Here's how the part is built. I have some questions about the finished solid (model axes, mm). Face numbers are marked on the shaded views. A direction names the side the tool comes from. Round coordinates to 2 decimals unless told otherwise and drop trailing zeros. Write each loop counter-clockwise with the first axis right and the second up, starting at its lowest first coordinate (ties: lowest second). Pieces come first, ordered by that corner, then holes. Notation, with made-up numbers: M 32,22 L 43,22 A26 ccw 43,46 Z; hole C 13,34 d10. An arc over 180 degrees is marked long. Write item = value, one per line. Start each with the question number.
(1) Will these pins go through, and if not, where does the flat tip stop? pin 1 Ø1 at (x, z) = (13.5, 1) entering from -Y; pin 2 Ø5 at (x, z) = (11, 3.5) entering from -Y; pin 3 Ø2 at (x, z) = (13, 0.5) entering from +Y.
(2) On a 3-axis mill with a long thin cutter (end or side, diameter ignored), from which of +Z, -Z, +X, -X, +Y, -Y can I reach the whole of each face in a straight line? I mean the marked faces 4 and 5. Say none if no direction works.
(3) I need wall thicknesses on line 1 along X through (y, z) = (-0.5, -4.25); line 2 along Z through (x, y) = (12.5, 0); line 3 along Z through (x, y) = (2.25, -1.5). Which ranges of each line are inside material? Lowest first, please.
(4) I want a section at B-B (x = 15). List the corners of the cut face in (y, z) for me, and give its area (3 significant figures).
(5) I want a section at A-A (z = 0). List the corners of the cut face in (x, y) for me.
(6) If we mould it in two halves opening along Z, with no side actions, what happens to the marked faces 1, 2 and 3? For each: released by +Z, released by -Z, zero draft, split by the parting line, or undercut.
```python
from build123d import *

# Parameters (mm, degrees)
CUT_EXTRUDE_1_DEPTH = 2.5
FILLET_1_R          = 0.3
CHAMFER_1_SIZE      = 1


with BuildPart() as part:
    # Эскиз1 → Повернуть1 (revolve)
    with BuildSketch(Plane.XY):
        Polygon((0, 0), (0, 5), (6, 5), (6, 3), (18, 3), (18, 0), align=None)
    revolve(axis=Axis((18, 0, 0), (-1, 0, 0)))

    # Эскиз2 → Вырез-Вытянуть1 (cut)
    with BuildSketch(Plane.ZY):
        Polygon((-1.443375673, 2.5), (-2.886751346, 0), (-1.443375673, -2.5), (1.443375673, -2.5), (2.886751346, 0), (1.443375673, 2.5), align=None)
    extrude(amount=-CUT_EXTRUDE_1_DEPTH, mode=Mode.SUBTRACT)

    # Скругление1
    fillet_1_edges = [part.edges().sort_by_distance(p)[0] for p in [
        (6, -3, 0),
        (0, -5, 0),
    ]]
    fillet(fillet_1_edges, radius=FILLET_1_R)

    # Фаска1
    chamfer_1_edges = [part.edges().sort_by_distance(p)[0] for p in [
        (18, -3, 0),
    ]]
    chamfer(chamfer_1_edges, length=CHAMFER_1_SIZE)


solid = part.part
```
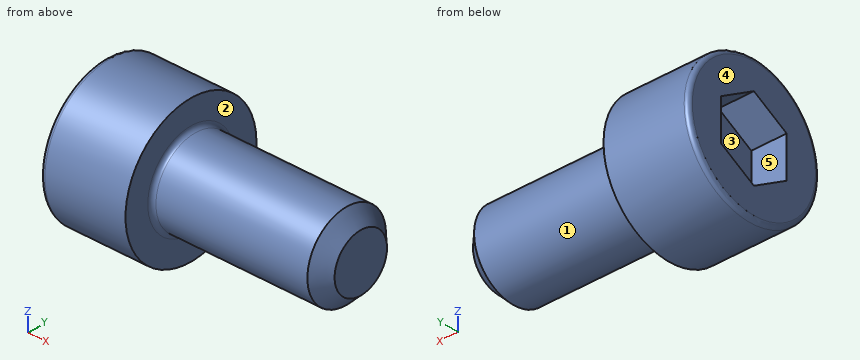
Returned:
q1.pin_1 = -2.96
q1.pin_2 = -2.83
q1.pin_3 = 3
q2.face_4 = +Z, -Z, -X, +Y, -Y
q2.face_5 = -X
q3.line_1 = 0 to 6
q3.line_2 = -3 to 3
q3.line_3 = -4.77 to -2.02, 2.02 to 4.77
q4.outline = C 0,0 d6
q4.area = 28.3 mm²
q5.outline = M 0,-4.7 A0.3 ccw 0.3,-5 L 6,-5 L 6,-3.3 A0.3 cw 6.3,-3 L 17,-3 L 18,-2 L 18,2 L 17,3 L 6.3,3 A0.3 cw 6,3.3 L 6,5 L 0.3,5 A0.3 ccw 0,4.7 L 0,2.5 L 2.5,2.5 L 2.5,-2.5 L 0,-2.5 Z
q6.face_1 = split by the parting line
q6.face_2 = zero draft
q6.face_3 = undercut
